Autodesk Inventor part; units mm, degrees
ref_plane "YZ Plane" through (0, 0, 0) normal (1, 0, 0) x (0, 1, 0)
ref_plane "XZ Plane" through (0, 0, 0) normal (0, 1, 0) x (-1, 0, 0)
ref_plane "XY Plane" through (0, 0, 0) normal (0, 0, 1) x (1, 0, 0)
sketch "Sketch2" plane through (0, 0, 0) normal (0, 0, 1) x (1, 0, 0)
  line L0 (-53, -88.9) -> (53, -88.9)
  line L1 (53, -88.9) -> (53, 88.9)
  line L2 (53, 88.9) -> (-53, 88.9)
  line L3 (-53, 88.9) -> (-53, -88.9)
  line L4 (-53, -88.9) -> (53, 88.9) construction
  line L5 (53, -88.9) -> (-53, 88.9) construction
  point P0 (0, 0)
  dimension "d0" = 106
  dimension "d1" = 177.8
extrude "Extrusion1" add sketch "Sketch2" against normal blind 6.35
sketch "Sketch5" plane through (0, 0, 0) normal (0, 0, 1) x (1, 0, 0)
  circle A0 centre (0, 0) radius 25.4
  dimension "d26" = 50.8
extrude "CenterHole" cut sketch "Sketch5" against normal through all
sketch "Sketch6" plane through (0, 0, 0) normal (0, 0, 1) x (1, 0, 0)
  line L0 (-53, 88.9) -> (-53, -88.9)
  line L1 (53, -88.9) -> (53, 88.9)
  line L2 (-53, -88.9) -> (-53, 88.9) construction
  line L3 (-53, 82.4) -> (53, 82.4) construction
  line L4 (53, 88.9) -> (-53, 88.9) construction
  point P0 (0, 0)
  point P1 (0, 82.4)
  point P2 (123.3454, 23.3667)
  point P3 (-25, 82.4)
  point P4 (25, 82.4)
  dimension "d29" = 6.5
  dimension "d30" = 25
  dimension "d31" = 25
hole "TopThreeHoles" at (0, 82.4, 0) at (123.3454, 23.3667, 0) at (-25, 82.4, 0) at (25, 82.4, 0) direction (0, 0, -1) diameter 2.6416 end through all
sketch "Sketch7" plane through (0, 0, 0) normal (0, 0, 1) x (1, 0, 0)
  line L0 (53, -88.9) -> (53, 88.9)
  line L1 (-53, 88.9) -> (-53, -88.9)
  line L2 (-53, -37.1) -> (53, -37.1) construction
  line L3 (53, 88.9) -> (53, -88.9)
  line L4 (53, 88.9) -> (-53, 88.9) construction
  point P0 (0, 0)
  point P1 (-48, -37.1)
  point P2 (48, -37.1)
  dimension "d39" = 126
  dimension "d40" = 5
  dimension "d41" = 5
hole "Hole3" at (-48, -37.1, 0) at (48, -37.1, 0) direction (0, 0, -1) diameter 2.6416 end through all
properties part number "gateGasket"
Read the model definition and answer for the solid it produces. Units are mm, in the model's axes. Coordinates: 2 decimals unless noted, no trailing zeros. Loops run counter-clockwise (first coordinate to the right, second up) from the corner with the lowest first, then second, coordinate; pieces in that order, holes last. Notation, with made-up numbers: (89.5, 3) - (114.5, 3) arc R24 cw to (114.5, 30) - close; hole circle Ø5 at (76, 77.5). An arc over 180 degrees is marked (long way). Answer in a Markdown table with one row per item.
Q1. Find section A-A on y = 0. Write down the section's boundary in (x, z).
Here are the results:
| item | result |
|---|---|
| outline | (-53, -6.35) - (-25.4, -6.35) - (-25.4, 0) - (-53, 0) - close; (25.4, -6.35) - (53, -6.35) - (53, 0) - (25.4, 0) - close |
Q2. Straight lines are drawn through the part: line 1 along Y through (x, z) = (0, -4.25); line 2 along X through (y, z) = (-37.1, -3.5); line 3 along X through (y, z) = (82.4, -4.5). For each, find the intervals that lie inside material, in ascending order. Write a range as [from, to].
Here are the results:
| item | result |
|---|---|
| line 1 | y = [-88.9, -25.4], [25.4, 81.08], [83.72, 88.9] |
| line 2 | x = [-53, -49.32], [-46.68, 46.68], [49.32, 53] |
| line 3 | x = [-53, -26.32], [-23.68, -1.32], [1.32, 23.68], [26.32, 53] |
Q3. Find section B-B on z = -3.25. Write down the section's boundary in (x, y).
Here are the results:
| item | result |
|---|---|
| outline | (-53, -88.9) - (53, -88.9) - (53, 88.9) - (-53, 88.9) - close; hole circle Ø2.64 at (-48, -37.1); hole circle Ø2.64 at (-25, 82.4); hole circle Ø50.8 at (0, 0); hole circle Ø2.64 at (0, 82.4); hole circle Ø2.64 at (25, 82.4); hole circle Ø2.64 at (48, -37.1) |
Q4. Find section C-C on x = 16. Write down the section's boundary in (y, z), plus the area to 3 significant figures.
Here are the results:
| item | result |
|---|---|
| outline | (-88.9, -6.35) - (-19.73, -6.35) - (-19.73, 0) - (-88.9, 0) - close; (19.73, -6.35) - (88.9, -6.35) - (88.9, 0) - (19.73, 0) - close |
| area | 878 mm^2 |
Q5. The mould has two halves that part along X. Classify faces 1 (the flat face through (1, 88.9, -3)), 2 (the cylindrical face through (-5.506, -24.796, -3.131)), 3 (the flat face through (-53, 1, -3)): pulls with the +X half, pulls with the -X half, needs draft (parallel to the pull), parting line crosses it, or undercut.
Here are the results:
| item | result |
|---|---|
| face 1 | needs draft |
| face 2 | undercut |
| face 3 | pulls with the -X half |
